Can you work these out from the drawing? Everything is in mm from the part's minimum corner. A direction names the side the tool comes from. Give positions to 0.01 mm unless a question says otherwise; leave off trailing zeros. Loops run counter-clockwise (first coordinate to the right, second up) from the corner with the lowest first, then second, coordinate; pieces in that order, holes last.
Q1. If we section it at C-C (x = 86.04): Please give me the cut outline in (y, z), plus the area to 3 significant figures.
Q2. Will these pins go through, and if not, where does the flat tip stop? P1, Ø2, axis at x = 71.5, z = 1.5, coming from the -Y side; P2, Ø1.5, axis at x = 28.5, y = 38, coming from the +Z side; P3, Ø6, axis at x = 13.5, z = 16, coming from the +Y side.
Q3. If we section it at D-D (x = 115): Please give me the cut outline in (y, z).
Q4. If we section it at A-A (z = 14): Please give me the cut outline in (x, y).
Q5. If we section it at B-B (y = 32.62): Please give me the cut outline in (x, z), plus the area to 3 significant figures.
Q6. For the marked faces 1 and 2, which set-ups out of +Z, -Z, +X, -X, +Y, -Y let a thin tool reach every point of the face, with its end or its side?
Q7. I need wall thicknesses on line 1 (X direction, y = 2, z = 34); line 2 (Y direction, x = 86.04, z = 3.1); line 3 (Z direction, x = 120, y = 2). Which ranges of each line are inside material? Lowest first, please.
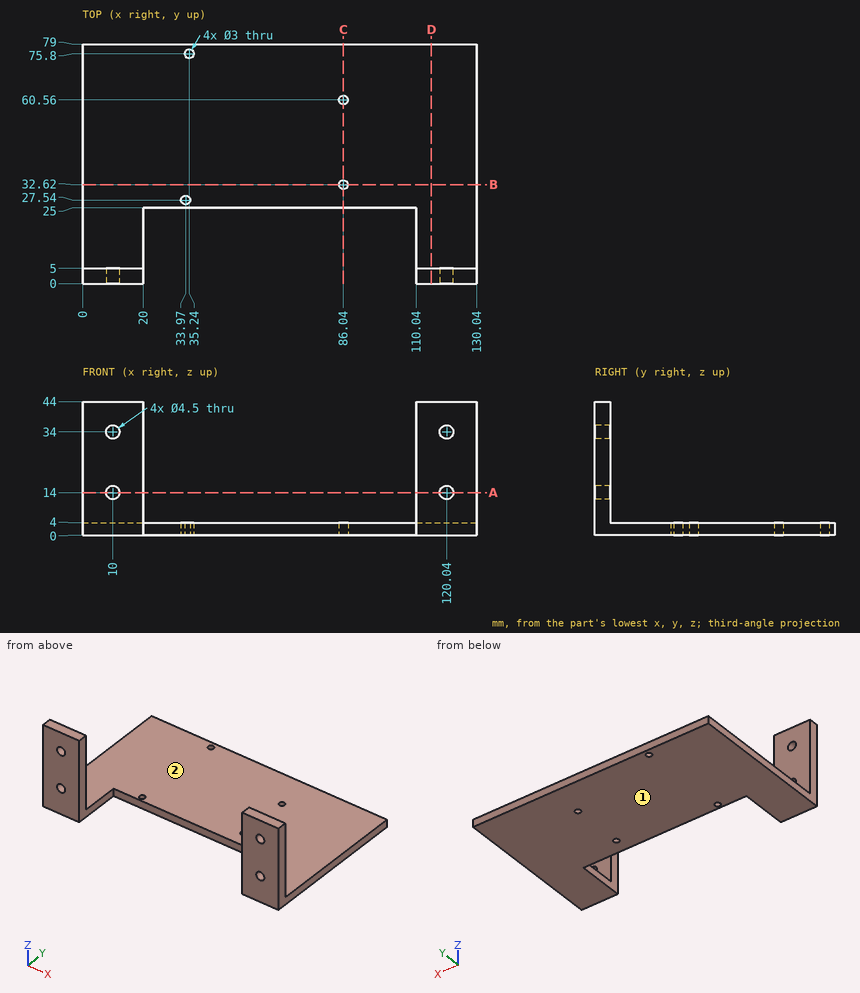
Check sheet entries:
1. outline: (25, 0) - (31.12, 0) - (31.12, 4) - (25, 4) - close; (34.12, 0) - (59.06, 0) - (59.06, 4) - (34.12, 4) - close; (62.06, 0) - (79, 0) - (79, 4) - (62.06, 4) - close
1. area: 192 mm2
2. P1: stops at y = 25
2. P2: stops at z = 4
2. P3: stops at y = 5
3. outline: (0, 0) - (79, 0) - (79, 4) - (5, 4) - (5, 44) - (0, 44) - close
4. outline: (0, 0) - (7.75, 0) - (7.75, 5) - (0, 5) - close; (12.25, 0) - (20, 0) - (20, 5) - (12.25, 5) - close; (110.04, 0) - (117.79, 0) - (117.79, 5) - (110.04, 5) - close; (122.29, 0) - (130.04, 0) - (130.04, 5) - (122.29, 5) - close
5. outline: (0, 0) - (84.54, 0) - (84.54, 4) - (0, 4) - close; (87.54, 0) - (130.04, 0) - (130.04, 4) - (87.54, 4) - close
5. area: 508 mm2
6. face 1: -Z, +X, -X, +Y, -Y
6. face 2: +Z, +X, -X, +Y
7. line 1: x = 0 to 7.75, 12.25 to 20, 110.04 to 117.79, 122.29 to 130.04
7. line 2: y = 25 to 31.12, 34.12 to 59.06, 62.06 to 79
7. line 3: z = 0 to 11.75, 16.25 to 31.75, 36.25 to 44
